The model under review builds one solid part; all positions refer to its coordinate system, in mm. A direction names the side the tool comes from. Round coordinates to 2 decimals unless told otherwise and drop trailing zeros. Write each loop counter-clockwise with the first axis right and the second up, starting at its lowest first coordinate (ties: lowest second). Pieces come first, ordered by that corner, then holes. Notation, with made-up numbers: M 40,-34 L 68,-34 A14 cw 68,-12 Z; hole C 27,14 d2. An arc over 180 degrees is marked long. One line per item, written item: value. Start each with the question number.
1) For P1, Ø4, axis at x = 4.5, z = -9.5, coming from the +Y side; P2, Ø2.5, axis at y = 2.5, z = -15.27, coming from the -X side; P3, Ø2, axis at y = 2.5, z = -15.27, coming from the +X side, all flat-tipped, find the tip position at first contact; note any pin that passes through.
2) Take a section at B-B, the plane z = -1.5. Write out the cut boundary in (x, y).
3) Take a section at D-D, the plane z = 12. Write out the cut boundary in (x, y).
4) Take a section at C-C, the plane x = 22.75. Write out the cut boundary in (y, z).
5) Wall thickness on probe 1 along Z at (x, y) = (49.05, 2.5); probe 2 along X at (y, z) = (4.4, 15); probe 3 along X at (y, z) = (0.95, 17.5): over which ranges is each line inside the solid? List them lowest first.
6) Mouldability with a two-part tool opening along X and no side actions: class faces 5 (the face through (10, 5, -11)), 6 (the face through (48.026, 2, 18)), 7 (the face through (-51.234, 2, 1)) as +X half, -X half, draft (parallel to the pull), parting line (faces both ways), or undercut.
7) Tool access review of faces 1 (the face through (-1, 2, 25.234)), 2 (the face through (49.376, 3.143, 17.286)), 3 (the face through (-38.71, 1.48, -16.6)), 4 (the face through (47, 2, -11.866)): name each direction out of +Z, -Z, +X, -X, +Y, -Y from which nothing blocks a thin tool from reaching the whole face with its end or side.
8) Take a section at A-A, the plane x = 39. Write out the cut boundary in (y, z), and give its area (3 significant figures).
from build123d import *

# Parameters (mm, degrees)
AGUJEROS_W          = 101.999998093
AGUJEROS_H          = 49.999999814
AGUJEROS_R          = 10.000041491
AGUJEROS_R_2        = 14.000010245
AGUJEROS_R_3        = 10.000041173
AGUJEROS_W_2        = 2.599999308
AGUJEROS_H_2        = 5.899999291
AGUJEROS_W_3        = 2.599999309
BOSS_EXTRUDE1_DEPTH = 5
BASE_R              = 1.72
CUT_EXTRUDE1_DEPTH  = 58.330053722
SKETCH4_R           = 1.68
CUT_EXTRUDE2_DEPTH  = 20
CUT_EXTRUDE3_START  = -20
AGUJEROSLATERALES_R = 1.68
CUT_EXTRUDE3_DEPTH  = 20


with BuildPart() as part:
    # Agujeros → Boss-Extrude1 (new body)
    with BuildSketch(Plane(origin=(0, 0, 0), x_dir=(1, 0, 0), z_dir=(0, 1, 0))):
        with Locations((-0.234376955, -0.234376955)):
            Rectangle(AGUJEROS_W, AGUJEROS_H)
        with Locations(Location((31.765623825, -0.234375367, 0), (0, 0, 270))):
            Circle(AGUJEROS_R, mode=Mode.SUBTRACT)
        with Locations(Location((-0.234386768, -0.23435079, 0), (0, 0, 270))):
            Circle(AGUJEROS_R_2, mode=Mode.SUBTRACT)
        with Locations(Location((-32.23437504, -0.234378061, 0), (0, 0, 270))):
            Circle(AGUJEROS_R_3, mode=Mode.SUBTRACT)
        with Locations((46.725622994, -16.184378266)):
            Rectangle(AGUJEROS_W_2, AGUJEROS_H_2, mode=Mode.SUBTRACT)
        with Locations((46.725622994, 14.815623091)):
            Rectangle(AGUJEROS_W_2, AGUJEROS_H_2, mode=Mode.SUBTRACT)
        with Locations((-47.274377513, -16.184378266)):
            Rectangle(AGUJEROS_W_3, AGUJEROS_H_2, mode=Mode.SUBTRACT)
        with Locations((-47.274377513, 14.815623091)):
            Rectangle(AGUJEROS_W_3, AGUJEROS_H_2, mode=Mode.SUBTRACT)
    extrude(amount=BOSS_EXTRUDE1_DEPTH)

    # Base → Cut-Extrude1 (cut, through all)
    with BuildSketch(Plane(origin=(0, 5, 0), x_dir=(1, 0, 0), z_dir=(0, 1, 0))):
        with Locations(Location((0, 17.5, 0), (0, 0, 270))):
            Circle(BASE_R)
        with Locations(Location((-22.75, 17.5, 0), (0, 0, 270))):
            Circle(BASE_R)
        with Locations(Location((22.75, 17.5, 0), (0, 0, 270))):
            Circle(BASE_R)
        with Locations(Location((0, -17.5, 0), (0, 0, 270))):
            Circle(BASE_R)
        with Locations(Location((22.75, -17.5, 0), (0, 0, 270))):
            Circle(BASE_R)
        with Locations(Location((-22.75, -17.5, 0), (0, 0, 270))):
            Circle(BASE_R)
    extrude(amount=-CUT_EXTRUDE1_DEPTH, mode=Mode.SUBTRACT)

    # Sketch4 → Cut-Extrude2 (cut)
    with BuildSketch(Plane.ZY.offset(51.234376001)):
        with Locations((-15.265622952, 2.5)):
            Circle(SKETCH4_R)
        with Locations((15.734376862, 2.5)):
            Circle(SKETCH4_R)
    extrude(amount=-CUT_EXTRUDE2_DEPTH, mode=Mode.SUBTRACT)

    # AgujerosLaterales → Cut-Extrude3 (cut)
    with BuildSketch(Plane(origin=(50.765622092, 0, 0), x_dir=(0, 0, -1), z_dir=(1, 0, 0)).offset(CUT_EXTRUDE3_START)):
        with Locations(Location((-15.734376862, 2.5, 0), (0, 0, 180))):
            Circle(AGUJEROSLATERALES_R)
        with Locations(Location((15.265622952, 2.5, 0), (0, 0, 180))):
            Circle(AGUJEROSLATERALES_R)
    extrude(amount=CUT_EXTRUDE3_DEPTH, mode=Mode.SUBTRACT)


solid = part.part
Checked values:
1. P1: passes through
1. P2: stops at x = -31.23
1. P3: stops at x = 30.77
2. outline: M -51.23,0 L -42.08,0 L -42.08,5 L -51.23,5 Z; M -22.39,0 L -14.13,0 L -14.13,5 L -22.39,5 Z; M 13.66,0 L 21.92,0 L 21.92,5 L 13.66,5 Z; M 41.61,0 L 50.77,0 L 50.77,5 L 41.61,5 Z
3. outline: M -51.23,0 L -7.82,0 L -7.82,5 L -51.23,5 Z; M 7.35,0 L 50.77,0 L 50.77,5 L 7.35,5 Z
4. outline: M 0,-24.77 L 5,-24.77 L 5,-19.22 L 0,-19.22 Z; M 0,-15.78 L 5,-15.78 L 5,-4.09 L 0,-4.09 Z; M 0,4.56 L 5,4.56 L 5,15.78 L 0,15.78 Z; M 0,19.22 L 5,19.22 L 5,25.23 L 0,25.23 Z
5. probe 1: z = -24.77 to -16.95, -13.59 to 14.05, 17.41 to 25.23
5. probe 2: x = -51.23 to -48.57, -45.97 to 45.43, 48.03 to 50.77
5. probe 3: x = -51.23 to -48.57, -45.97 to -24.47, -21.03 to -1.72, 1.72 to 21.03, 24.47 to 45.43, 48.03 to 50.77
6. face 5: draft
6. face 6: undercut
6. face 7: -X half
7. face 1: +Z, +X, -X, +Y, -Y
7. face 2: +X
7. face 3: -X
7. face 4: +Y, -Y
8. outline: M 0,-24.77 L 5,-24.77 L 5,-6.67 L 0,-6.67 Z; M 0,7.14 L 5,7.14 L 5,25.23 L 0,25.23 Z; hole C 2.5,-15.27 d3.36; hole C 2.5,15.73 d3.36
8. area: 163 mm2
